Here's the drawing with two shaded views (mm, measured from the low corner). I have some questions. Round coordinates to 2 decimals unless told otherwise and drop trailing zeros. Write each loop counter-clockwise with the first axis right and the second up, starting at its lowest first coordinate (ties: lowest second). Pieces come first, ordered by that corner, then holes. Notation, with made-up numbers: M 65.25,85 L 116.25,85 A18 cw 116.25,113 Z; hole C 78.5,53 d2. An arc over 180 degrees is marked long. Write item = value, one per line. Start each with the question number.
(1) Will these pins go through, and if not, where does the flat tip stop? pin 1 Ø1 at (x, z) = (2.5, 3) entering from +Y; pin 2 Ø5 at (x, y) = (16.5, 16) entering from -Z; pin 3 Ø1.4 at (x, y) = (17, 10) entering from +Z; pin 4 Ø1.8 at (x, y) = (9.5, 10.5) entering from -Z.
(2) I need wall thicknesses on line 1 along Y through (x, z) = (10, 2.8); line 2 along Y through (x, z) = (10.5, 3.15); line 3 along Y through (x, z) = (10, 1.3). Which ranges of each line are inside material? Lowest first, please.
(3) I want a section at A-A (x = 10). List the corners of the cut face in (y, z) for me, and give its area (4 significant figures).
(4) I want a section at B-B (z = 2.8). List the corners of the cut face in (x, y) for me.
(5) If we mould it in two halves opening along X, with no side actions, what happens to the marked faces 1, 2 and 3? For each: released by +X, released by -X, zero draft, split by the parting line, or undercut.
(6) I want a section at C-C (y = 3). List the corners of the cut face in (x, z) for me, and give its area (3 significant figures).
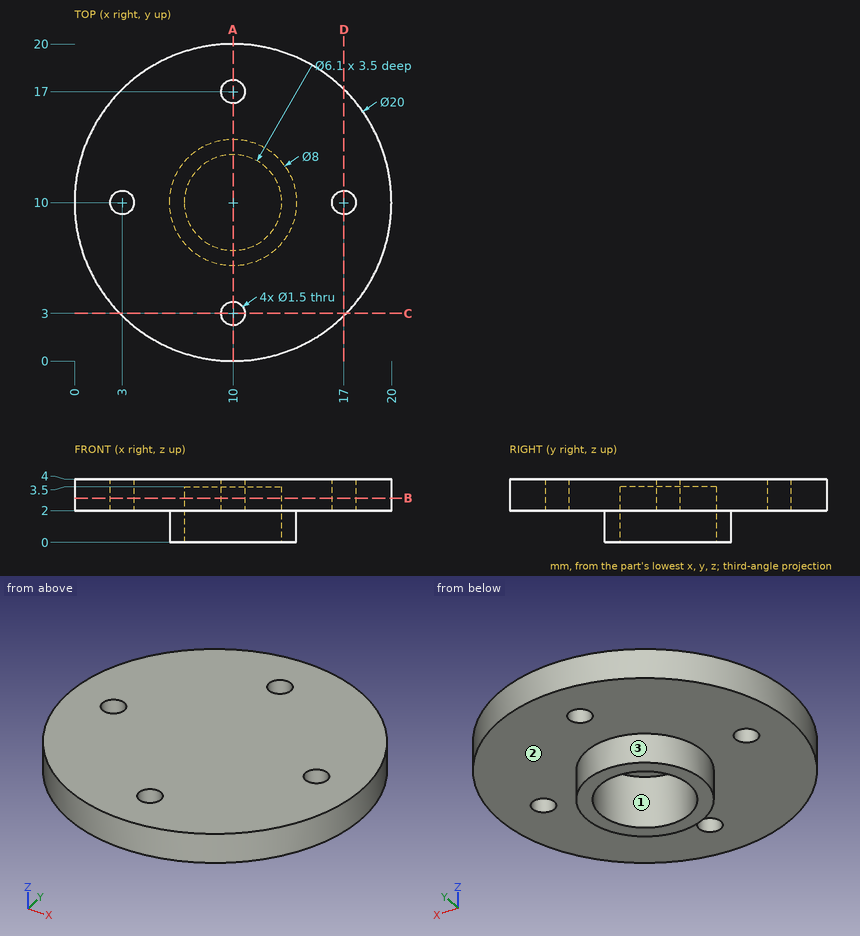
Returned:
q1.pin_1 = 17.14
q1.pin_2 = 2
q1.pin_3 = through
q1.pin_4 = 3.5
q2.line_1 = 0 to 2.25, 3.75 to 6.95, 13.05 to 16.25, 17.75 to 20
q2.line_2 = 0.01 to 2.44, 3.56 to 6.99, 13.01 to 16.44, 17.56 to 19.99
q2.line_3 = 6 to 6.95, 13.05 to 14
q3.outline = M 0,2 L 2.25,2 L 2.25,4 L 0,4 Z; M 3.75,2 L 6,2 L 6,0 L 6.95,0 L 6.95,3.5 L 13.05,3.5 L 13.05,0 L 14,0 L 14,2 L 16.25,2 L 16.25,4 L 3.75,4 Z; M 17.75,2 L 20,2 L 20,4 L 17.75,4 Z
q3.area = 28.65 mm²
q4.outline = C 10,10 d20; hole C 3,10 d1.5; hole C 10,10 d6.1; hole C 10,3 d1.5; hole C 10,17 d1.5; hole C 17,10 d1.5
q5.face_1 = undercut
q5.face_2 = zero draft
q5.face_3 = split by the parting line
q6.outline = M 2.86,2 L 9.25,2 L 9.25,4 L 2.86,4 Z; M 10.75,2 L 17.14,2 L 17.14,4 L 10.75,4 Z
q6.area = 25.6 mm²
